Read the model definition and answer for the solid it produces. Units are mm, in the model's axes. A direction names the side the tool comes from. Coordinates: 2 decimals unless noted, no trailing zeros. Order: outer loops, then holes, each group sorted by start corner. A loop starts at its lowest first (then second) coordinate and runs counter-clockwise, first axis right, second up. Notation, with made-up numbers: M 50.25,87 L 93.25,87 A22 cw 93.25,114 Z; hole C -38,-17.75 d5. An arc over 180 degrees is marked long. Use a Markdown table: item, result. Add a question column.
1) Find section C-C on y = 9.25. Write down the section's boundary in (x, z).
2) Each of these flat-tipped pins is pushed along its axis until it touches: pin 1 Ø1 at (y, z) = (0, 3) entering from +X; pin 2 Ø5 at (y, z) = (6, -0.5) entering from -X; pin 3 Ø1.2 at (x, z) = (0.5, 3.5) entering from -Y; pin 4 Ø3 at (x, y) = (0, 7.14) entering from -Z. Where does it stop, or does it pass through?
3) The mould has two halves that part along X. Classify faces 1 (the face through (7.696, -3.003, 2.791)), 2 (the face through (-11.984, 1.182, 2.788)), 3 (the face through (-1, 5, -3)): released by +X, released by -X, zero draft, split by the parting line, or undercut.
4) Find section A-A on x = 0. Write down the section's boundary in (y, z), plus the area to 3 significant figures.
5) For faces 4 (the face through (-2, 3, 0)), 5 (the face through (-3, 5.5, 3)), 6 (the face through (2.84, 18.37, 2.79)), determine the directions among +Z, -Z, +X, -X, +Y, -Y from which every point of the face is accessible in a straight line to the end or side of a thin tool.
6) Find section D-D on y = 4.75. Write down the section's boundary in (x, z).
7) Find the intervals of material crossed by probe 1 along Y at (x, z) = (0, -2); probe 2 along Y at (x, z) = (0.5, 4.75); probe 3 along X at (y, z) = (7.25, 5.25), in increasing order. Write a range as [from, to].
from build123d import *

# Parameters (mm, degrees)
BOSS_EXTRUDE1_DEPTH = 5.5
FILLET1_R           = 1
SKETCH2_R           = 4
BOSS_EXTRUDE2_DEPTH = 3
SKETCH3_R           = 1.75
CUT_EXTRUDE3_DEPTH  = 5
SKETCH4_R           = 1.75
CUT_EXTRUDE4_DEPTH  = 9.5000001


with BuildPart() as part:
    # Sketch1 → Boss-Extrude1 (new body)
    with BuildSketch(Plane.XY):
        with BuildLine():
            Line((-3.860140394, 18.642037645), (3.139859606, 18.642037645))
            ThreePointArc((3.139859606, 18.642037645), (5.695506545, 8.64046477), (12.898136912, 1.245540359))
            Line((12.898136912, 1.245540359), (7.648136912, -3.384524435))
            ThreePointArc((7.648136912, -3.384524435), (0.148136912, 0.001097287), (-7.351863088, -3.384524435))
            Line((-7.351863088, -3.384524435), (-12.601863088, 1.245540359))
            ThreePointArc((-12.601863088, 1.245540359), (-5.871247517, 8.758014837), (-3.860140394, 18.642037645))
        make_face()
    extrude(amount=BOSS_EXTRUDE1_DEPTH)

    # Fillet1
    fillet1_edges = [part.edges().sort_by_distance(p)[0] for p in [
        (-3.860140394, 18.642037645, 2.75),
        (3.139859606, 18.642037645, 2.75),
        (12.898136912, 1.245540359, 2.75),
        (7.648136912, -3.384524435, 2.75),
        (-7.351863088, -3.384524435, 2.75),
        (-12.601863088, 1.245540359, 2.75),
        (10.273136912, -1.069492038, 0),
    ]]
    fillet(fillet1_edges, radius=FILLET1_R)

    # Sketch2 → Boss-Extrude2 (add)
    with BuildSketch(Plane(origin=(0, 0, 0), x_dir=(-1, 0, 0), z_dir=(0, 0, -1))):
        with Locations((0, 7.142037645)):
            Circle(SKETCH2_R)
    extrude(amount=BOSS_EXTRUDE2_DEPTH)

    # Sketch3 → Cut-Extrude3 (cut)
    with BuildSketch(Plane.XY.offset(5.5)):
        Polygon((-3.95, 7.142037645), (-1.975, 3.7212373), (1.975, 3.7212373), (3.95, 7.142037645), (1.975, 10.56283799), (-1.975, 10.56283799), align=None)
        with Locations((0, 7.142037645)):
            Circle(SKETCH3_R, mode=Mode.SUBTRACT)
    extrude(amount=-CUT_EXTRUDE3_DEPTH, mode=Mode.SUBTRACT)

    # Sketch4 → Cut-Extrude4 (cut, through all)
    with BuildSketch(Plane(origin=(0, 0, -3), x_dir=(-1, 0, 0), z_dir=(0, 0, -1))):
        with Locations((0, 7.142037645)):
            Circle(SKETCH4_R)
    extrude(amount=-CUT_EXTRUDE4_DEPTH, mode=Mode.SUBTRACT)


solid = part.part
Check result:
| question | item | result |
|---|---|---|
| 1 | outline | M -5.63,0 L -3.4,0 L -3.4,-3 L 3.4,-3 L 3.4,0 L 5.37,0 L 5.37,5.5 L 2.73,5.5 L 2.73,0.5 L -2.73,0.5 L -2.73,5.5 L -5.63,5.5 Z |
| 2 | pin 1 | stops at x = 12.03 |
| 2 | pin 2 | stops at x = -9.7 |
| 2 | pin 3 | stops at y = -0.04 |
| 2 | pin 4 | passes through |
| 3 | face 1 | undercut |
| 3 | face 2 | released by -X |
| 3 | face 3 | zero draft |
| 4 | outline | M 0,0 L 3.14,0 L 3.14,-3 L 5.39,-3 L 5.39,0.5 L 3.72,0.5 L 3.72,5.5 L 0,5.5 Z; M 8.89,-3 L 11.14,-3 L 11.14,0 L 18.64,0 L 18.64,5.5 L 10.56,5.5 L 10.56,0.5 L 8.89,0.5 Z |
| 4 | area | 80.1 mm2 |
| 5 | face 4 | -Z |
| 5 | face 5 | +Z |
| 5 | face 6 | +Z, -Z, +X, +Y |
| 6 | outline | M -8.56,0 L -3.21,0 L -3.21,-3 L 3.21,-3 L 3.21,0 L 8.54,0 L 8.54,5.5 L 2.57,5.5 L 2.57,0.5 L -2.57,0.5 L -2.57,5.5 L -8.56,5.5 Z |
| 7 | probe 1 | y = [3.14, 5.39], [8.89, 11.14] |
| 7 | probe 2 | y = [-0.01, 3.72], [10.56, 18.64] |
| 7 | probe 3 | x = [-6.72, -3.89], [3.89, 6.55] |
